```python
from build123d import *

# Parameters (mm, degrees)
SKETCH3_R           = 2.95
BOSS_EXTRUDE1_DEPTH = 83.4
SKETCH4_W           = 10
SKETCH4_H           = 10
BOSS_EXTRUDE2_DEPTH = 3


with BuildPart() as part:
    # Sketch3 → Boss-Extrude1 (new body)
    with BuildSketch(Plane(origin=(0, 0, 0), x_dir=(0, 0, -1), z_dir=(1, 0, 0))):
        Circle(SKETCH3_R)
    extrude(amount=-BOSS_EXTRUDE1_DEPTH)

    # Sketch4 → Boss-Extrude2 (add)
    with BuildSketch(Plane(origin=(0, 0, 0), x_dir=(0, 0, -1), z_dir=(1, 0, 0))):
        Rectangle(SKETCH4_W, SKETCH4_H)
    extrude(amount=BOSS_EXTRUDE2_DEPTH)


solid = part.part
```
The listing builds one solid part. Answer for the finished solid, in the listing's coordinates (mm). A direction names the side the tool comes from. Round coordinates to 2 decimals unless told otherwise and drop trailing zeros. Order: outer loops, then holes, each group sorted by start corner. A loop starts at its lowest first (then second) coordinate and runs counter-clockwise, first axis right, second up. Notation, with made-up numbers: (-18, 69.25) - (32, 69.25) arc R20 cw to (32, 92.25) - close; hole circle Ø2 at (-36.75, 64). An arc over 180 degrees is marked (long way). Put each result on its own line as item: value. Start each with the question number.
(1) Given P1, Ø1.5, axis at x = -14, y = -1.5, coming from the -Z side; P2, Ø2, axis at x = -43, z = -1.5, coming from the +Y side; P3, Ø6, axis at y = 0.5, z = 3, coming from the -X side; P4, Ø3, axis at x = -24.5, z = -2, coming from the -Y side, each flat-ended and moving along its own axis, determine where each tip first touches the part or whether it passes through.
(2) For faces 1 (the flat face through (0, 2.3, -2.2)), 2 (the flat face through (1, 0, 5)), determine the directions among +Z, -Z, +X, -X, +Y, -Y from which every point of the face is accessible in a straight line to the end or side of a thin tool.
(3) Find section A-A (z = 0). Give the vertices of the cut face in (x, y).
(4) Find section C-C (x = -18.5). Give the vertices of the cut face in (y, z), plus the area to 3 significant figures.
(5) Straight lines are drawn through the part: probe 1 along X at (y, z) = (0.75, 3); probe 2 along Y at (x, z) = (-64, -2). For each, find the intervals that lie inside material, in ascending order. Write a range as from..to.
Reply:
1. P1: z = -2.85
1. P2: y = 2.91
1. P3: x = -83.4
1. P4: y = -2.91
2. face 1: -X
2. face 2: +Z, +X, -X, +Y, -Y
3. outline: (-83.4, -2.95) - (0, -2.95) - (0, -5) - (3, -5) - (3, 5) - (0, 5) - (0, 2.95) - (-83.4, 2.95) - close
4. outline: circle Ø5.9 at (0, 0)
4. area: 27.3 mm^2
5. probe 1: 0..3
5. probe 2: -2.17..2.17
